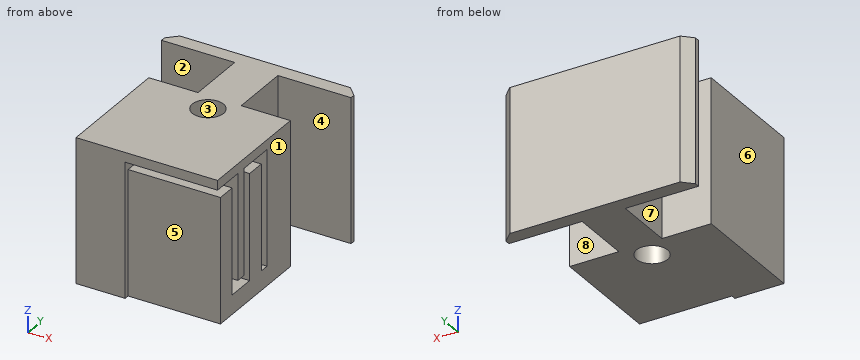
```python
from build123d import *

# Parameters (mm, degrees)
BOSS_EXTRUDE1_DEPTH          = 30
SKETCH2_R                    = 3.25
CUT_EXTRUDE1_DEPTH           = 36
CUT_EXTRUDE_THIN1_DEPTH      = 62.144173884
CUT_EXTRUDE_THIN1_DEPTH_BACK = 19.25
CHAMFER2_SIZE                = 2


with BuildPart() as part:
    # Sketch1 → Boss-Extrude1 (new body)
    with BuildSketch(Plane.XY):
        Polygon((0, 0), (-10.25, 0), (-15.25, 0), (-15.25, -3), (-10.25, -3), (0, -3), (0, -15.6), (-10.25, -15.6), (-10.25, -40.6), (19.25, -40.6), (19.25, -15.6), (9, -15.6), (9, -3), (19.25, -3), (24.25, -3), (24.25, 0), (19.25, 0), (9, 0), align=None)
    extrude(amount=BOSS_EXTRUDE1_DEPTH)

    # Sketch2 → Cut-Extrude1 (cut)
    with BuildSketch(Plane.XY.offset(30)):
        with Locations((4.5, -19.6)):
            Circle(SKETCH2_R)
    extrude(amount=-CUT_EXTRUDE1_DEPTH, mode=Mode.SUBTRACT)

    # Sketch3 → Cut-Extrude-Thin1 (cut, two sides: drawn at the far end of the back side and taken through both)
    with BuildSketch(Plane(origin=(19.25, 0, 0), x_dir=(0, 0, -1), z_dir=(1, 0, 0)).offset(-CUT_EXTRUDE_THIN1_DEPTH_BACK)):
        Polygon((0, -39.6), (-26, -39.6), (-26, -35.6), (-4, -35.6), (-4, -29.6), (-26, -29.6), (-26, -25.6), (-4, -25.6), (-4, -23.6), (-28, -23.6), (-28, -31.6), (-6, -31.6), (-6, -33.6), (-28, -33.6), (-28, -41.6), (0, -41.6), align=None)
    extrude(amount=CUT_EXTRUDE_THIN1_DEPTH + CUT_EXTRUDE_THIN1_DEPTH_BACK, mode=Mode.SUBTRACT)

    # Chamfer2
    chamfer2_edges = [part.edges().sort_by_distance(p)[0] for p in [
        (24.25, 0, 15),
        (-15.25, 0, 15),
    ]]
    chamfer(chamfer2_edges, length=CHAMFER2_SIZE)


solid = part.part
```
Model file for the job. Use its own axes, mm. Face numbers are marked on the shaded views. A direction names the side the tool comes from. Round coordinates to 2 decimals unless told otherwise and drop trailing zeros. Order: outer loops, then holes, each group sorted by start corner. A loop starts at its lowest first (then second) coordinate and runs counter-clockwise, first axis right, second up. Notation, with made-up numbers: M -11,12.5 L 19,12.5 A21 cw 19,49.5 Z; hole C 27,53.5 d11. An arc over 180 degrees is marked long. Use CSV: the item, a comma, the result in double quotes.
Item 1: Pin check, flat tips, straight feed: pin 1 (5 mm diameter, centred on y = -31, z = 14.5, fed in from +X); pin 2 (15.5 mm diameter, centred on x = 9, z = 13, fed in from -Y); pin 3 (1.5 mm diameter, centred on y = -34.5, z = 18, fed in from -X). Stop position of each tip, or through.
Worked answers:
pin 1,"x = 19.25"
pin 2,"y = -39.6"
pin 3,"x = -10.25"
Item 2: Saw through at B-B (y = -19.6). List the corners of the cut face in (x, z).
Worked answers:
outline,"M -10.25,0 L 1.25,0 L 1.25,30 L -10.25,30 Z; M 7.75,0 L 19.25,0 L 19.25,30 L 7.75,30 Z"
Item 3: Saw through at D-D (x = -7.5). List the corners of the cut face in (y, z).
Worked answers:
outline,"M -40.6,0 L -15.6,0 L -15.6,30 L -40.6,30 Z; M -3,0 L 0,0 L 0,30 L -3,30 Z"
Item 4: Which spindle directions (+Z, -Z, +X, -X, +Y, -Y) get a long thin tool onto all of the face, cutting with end or side? Do the marked faces 1, 2, 3 and 4. Say none if no direction does.
Worked answers:
face 1,"+Z, -Z, +X, -Y"
face 2,"+Z, -Z, -X"
face 3,"+Z, -Z"
face 4,"+Z, -Z, +X"
Item 5: Saw through at A-A (x = 4.5). List the corners of the cut face in (y, z).
Worked answers:
outline,"M -40.6,28 L -33.6,28 L -33.6,6 L -31.6,6 L -31.6,28 L -23.6,28 L -23.6,4 L -25.6,4 L -25.6,26 L -29.6,26 L -29.6,4 L -35.6,4 L -35.6,26 L -39.6,26 L -39.6,0 L -22.85,0 L -22.85,30 L -40.6,30 Z; M -16.35,0 L 0,0 L 0,30 L -16.35,30 Z"
Item 6: Pull direction Y, two halves, no side cores. Call the marked faces 5, 6, 7 and 8: released by +Y, released by -Y, zero draft, split by the parting line, or undercut.
Worked answers:
face 5,"released by -Y"
face 6,"zero draft"
face 7,"undercut"
face 8,"undercut"
Item 7: Probe probe 1 along Y at (x, z) = (4.5, 15.75); probe 2 along Y at (x, z) = (12, 19); probe 3 along Z at (x, y) = (1.5, -34). List the from-to ranges inside material, lowest first.
Worked answers:
probe 1,"-39.6 to -35.6, -33.6 to -31.6, -29.6 to -25.6, -23.6 to -22.85, -16.35 to 0"
probe 2,"-39.6 to -35.6, -33.6 to -31.6, -29.6 to -25.6, -23.6 to -15.6, -3 to 0"
probe 3,"0 to 4, 28 to 30"
